from build123d import *

# Parameters (mm, degrees)
SKETCH1_R           = 11.5
SKETCH1_R_2         = 1.75
BOSS_EXTRUDE1_DEPTH = 2
CHAMFER1_SIZE       = 0.25


with BuildPart() as part:
    # Sketch1 → Boss-Extrude1 (new body)
    with BuildSketch(Plane(origin=(0, 0, 0), x_dir=(1, 0, 0), z_dir=(0, 1, 0))):
        with BuildLine():
            Line((16.171038928, -21), (-16.171038928, -21))
            ThreePointArc((-16.171038928, -21), (-16.861657425, -20.876977915), (-17.467314594, -20.523046092))
            ThreePointArc((-17.467314594, -20.523046092), (-19.056527753, -19.056527753), (-20.523046092, -17.467314594))
            ThreePointArc((-20.523046092, -17.467314594), (-20.876977915, -16.861657425), (-21, -16.171038928))
            Line((-21, -16.171038928), (-21, 16.171038928))
            ThreePointArc((-21, 16.171038928), (-20.876977915, 16.861657425), (-20.523046092, 17.467314594))
            ThreePointArc((-20.523046092, 17.467314594), (-19.056527753, 19.056527753), (-17.467314594, 20.523046092))
            ThreePointArc((-17.467314594, 20.523046092), (-16.861657425, 20.876977915), (-16.171038928, 21))
            Line((-16.171038928, 21), (16.171038928, 21))
            ThreePointArc((16.171038928, 21), (16.861657425, 20.876977915), (17.467314594, 20.523046092))
            ThreePointArc((17.467314594, 20.523046092), (19.056527753, 19.056527753), (20.523046092, 17.467314594))
            ThreePointArc((20.523046092, 17.467314594), (20.876977915, 16.861657425), (21, 16.171038928))
            Line((21, 16.171038928), (21, -16.171038928))
            ThreePointArc((21, -16.171038928), (20.876977915, -16.861657425), (20.523046092, -17.467314594))
            ThreePointArc((20.523046092, -17.467314594), (19.056527753, -19.056527753), (17.467314594, -20.523046092))
            ThreePointArc((17.467314594, -20.523046092), (16.861657425, -20.876977915), (16.171038928, -21))
        make_face()
        with Locations(Location((0, 0, 0), (0, 0, 270))):
            Circle(SKETCH1_R, mode=Mode.SUBTRACT)
        with Locations(Location((15.5, -15.5, 0), (0, 0, 270))):
            Circle(SKETCH1_R_2, mode=Mode.SUBTRACT)
        with Locations(Location((15.5, 15.5, 0), (0, 0, 270))):
            Circle(SKETCH1_R_2, mode=Mode.SUBTRACT)
        with Locations(Location((-15.5, 15.5, 0), (0, 0, 270))):
            Circle(SKETCH1_R_2, mode=Mode.SUBTRACT)
        with Locations(Location((-15.5, -15.5, 0), (0, 0, 270))):
            Circle(SKETCH1_R_2, mode=Mode.SUBTRACT)
    extrude(amount=BOSS_EXTRUDE1_DEPTH)

    # Chamfer1
    chamfer1_edges = [part.edges().sort_by_distance(p)[0] for p in [
        (20.876977915, 2, 16.861657425),
        (21, 2, 0),
        (0, 0, 21),
        (-16.861657425, 0, 20.876977915),
        (-19.056527753, 0, 19.056527753),
        (-20.876977915, 0, 16.861657425),
        (-21, 0, 0),
        (20.876977915, 2, -16.861657425),
        (-20.876977915, 0, -16.861657425),
        (-19.056527753, 0, -19.056527753),
        (-16.861657425, 0, -20.876977915),
        (0, 0, -21),
        (16.861657425, 0, -20.876977915),
        (19.056527753, 0, -19.056527753),
        (20.876977915, 0, -16.861657425),
        (21, 0, 0),
        (19.056527753, 2, -19.056527753),
        (20.876977915, 0, 16.861657425),
        (19.056527753, 0, 19.056527753),
        (16.861657425, 0, 20.876977915),
        (16.861657425, 2, -20.876977915),
        (0, 2, -21),
        (-16.861657425, 2, -20.876977915),
        (-19.056527753, 2, -19.056527753),
        (-20.876977915, 2, -16.861657425),
        (-21, 2, 0),
        (0, 0, -11.5),
        (0, 2, -11.5),
        (16.861657425, 2, 20.876977915),
        (-20.876977915, 2, 16.861657425),
        (15.5, 0, 13.75),
        (15.5, 2, 13.75),
        (-19.056527753, 2, 19.056527753),
        (-16.861657425, 2, 20.876977915),
        (15.5, 0, -17.25),
        (15.5, 2, -17.25),
        (0, 2, 21),
        (-15.5, 0, -17.25),
        (-15.5, 2, -17.25),
        (-15.5, 0, 13.75),
        (-15.5, 2, 13.75),
        (19.056527753, 2, 19.056527753),
    ]]
    chamfer(chamfer1_edges, length=CHAMFER1_SIZE)


solid = part.part
Check sheet for the modelled part. Datum: model origin and axes. Units: mm. Round coordinates to 2 decimals unless told otherwise and drop trailing zeros. Order: outer loops, then holes, each group sorted by start corner. A loop starts at its lowest first (then second) coordinate and runs counter-clockwise, first axis right, second up.
(1) Draft check along Z on faces 1 (the cylindrical face through (20.88, 0.99, 16.85)), 2 (the cylindrical face through (-13.765, 0.99, 15.272)), 3 (the flat face through (-9, 0, 9)), 4 (the cylindrical face through (9.7, 0.99, 6.18)). Enter one of: pulls with the +Z half, pulls with the -Z half, needs draft (parallel to the pull), parting line crosses it, or undercut.
(2) Cross-section at B-B, the plane x = 15.5. Enter the section's corners in (y, z).
(3) Cross-section at A-A, the plane z = 0. Enter the section's corners in (x, y).
(4) Scan lines: probe 1 along X at (y, z) = (1, 15.5); probe 2 along Z at (x, y) = (16, 1.2); probe 3 along X at (y, z) = (0.85, 0). Record each from-to range of solid material in increasing order.
(5) Cross-section at C-C, the plane y = 1.2. Enter the section's corners in (x, z), and give its area (3 significant figures).
(6) Cross-section at D-D, the plane z = 15.5. Enter the section's corners in (x, y), and give its area (3 significant figures).
Check sheet entries:
1. face 1: pulls with the +Z half
1. face 2: undercut
1. face 3: needs draft
1. face 4: undercut
2. outline: (0, -20.75) - (0.25, -21) - (1.75, -21) - (2, -20.75) - (2, -17.5) - (1.75, -17.25) - (0.25, -17.25) - (0, -17.5) - close; (0, -13.5) - (0.25, -13.75) - (1.75, -13.75) - (2, -13.5) - (2, 13.5) - (1.75, 13.75) - (0.25, 13.75) - (0, 13.5) - close; (0, 17.5) - (0.25, 17.25) - (1.75, 17.25) - (2, 17.5) - (2, 20.75) - (1.75, 21) - (0.25, 21) - (0, 20.75) - close
3. outline: (-21, 0.25) - (-20.75, 0) - (-11.75, 0) - (-11.5, 0.25) - (-11.5, 1.75) - (-11.75, 2) - (-20.75, 2) - (-21, 1.75) - close; (11.5, 0.25) - (11.75, 0) - (20.75, 0) - (21, 0.25) - (21, 1.75) - (20.75, 2) - (11.75, 2) - (11.5, 1.75) - close
4. probe 1: x = -21 to -17.25, -13.75 to 13.75, 17.25 to 21
4. probe 2: z = -21 to -17.18, -13.82 to 13.82, 17.18 to 21
4. probe 3: x = -21 to -11.5, 11.5 to 21
5. outline: (-21, -16.17) arc R2 ccw to (-20.52, -17.47) arc R26.95 ccw to (-17.47, -20.52) arc R2 ccw to (-16.17, -21) - (16.17, -21) arc R2 ccw to (17.47, -20.52) arc R26.95 ccw to (20.52, -17.47) arc R2 ccw to (21, -16.17) - (21, 16.17) arc R2 ccw to (20.52, 17.47) arc R26.95 ccw to (17.47, 20.52) arc R2 ccw to (16.17, 21) - (-16.17, 21) arc R2 ccw to (-17.47, 20.52) arc R26.95 ccw to (-20.52, 17.47) arc R2 ccw to (-21, 16.17) - close; hole circle Ø3.5 at (-15.5, -15.5); hole circle Ø3.5 at (-15.5, 15.5); hole circle Ø23 at (0, 0); hole circle Ø3.5 at (15.5, -15.5); hole circle Ø3.5 at (15.5, 15.5)
5. area: 1,280 mm2
6. outline: (-21, 0.25) - (-20.75, 0) - (-17.5, 0) - (-17.25, 0.25) - (-17.25, 1.75) - (-17.5, 2) - (-20.75, 2) - (-21, 1.75) - close; (-13.75, 0.25) - (-13.5, 0) - (13.5, 0) - (13.75, 0.25) - (13.75, 1.75) - (13.5, 2) - (-13.5, 2) - (-13.75, 1.75) - close; (17.25, 0.25) - (17.5, 0) - (20.75, 0) - (21, 0.25) - (21, 1.75) - (20.75, 2) - (17.5, 2) - (17.25, 1.75) - close
6. area: 69.6 mm2
